Drawing for the job (mm, zero at the part's lowest x, y, z). Give positions to 0.01 mm unless a question says otherwise; leave off trailing zeros. Order: outer loops, then holes, each group sorted by start corner. A loop starts at its lowest first (then second) coordinate and runs counter-clockwise, first axis right, second up. Notation, with made-up numbers: (42.5, 48.5) - (66.5, 48.5) arc R15 ccw to (66.5, 52.5) - close; hole circle Ø7 at (-36, 44). An arc over 180 degrees is marked (long way). Use a Markdown table: item, result.
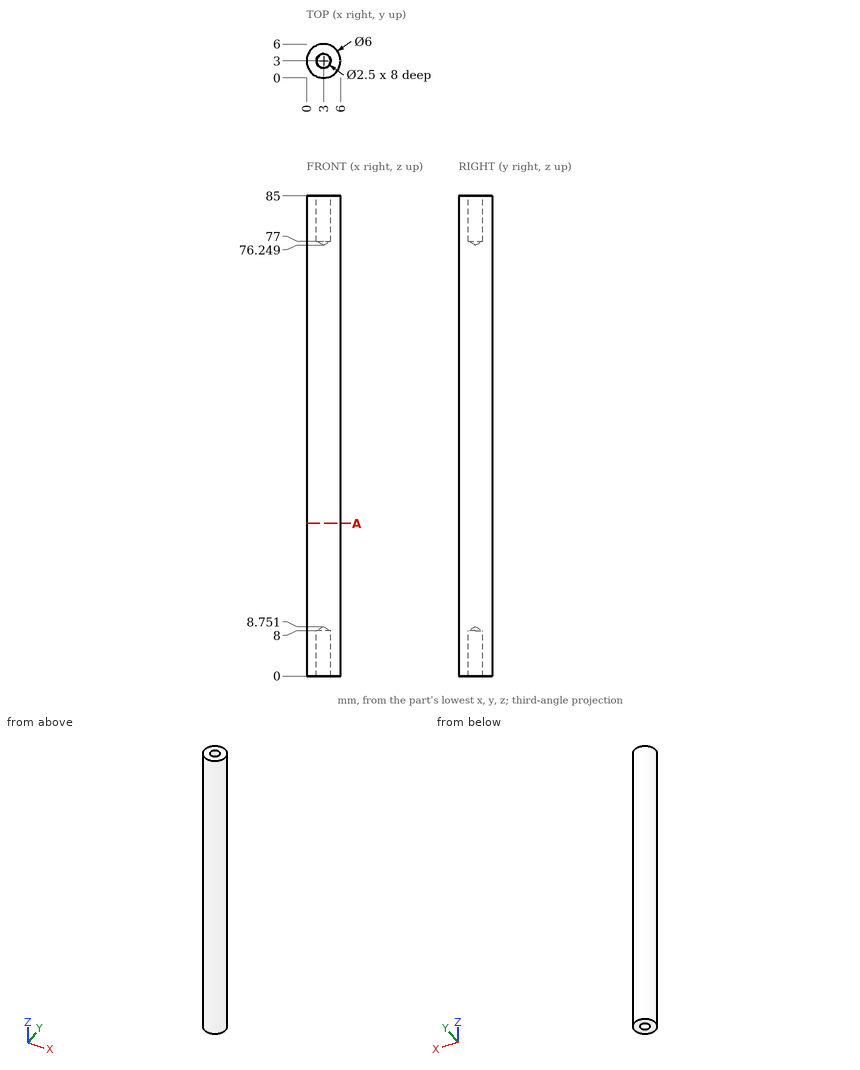
1) Wall check: line 1 (Y direction, x = 3, z = 4.25); line 2 (Y direction, x = 3.4, z = 54); line 3 (X direction, y = 4, z = 22). Give the ranges that are in metal, low to high. Write a range as from..to.
Computed:
| item | result |
|---|---|
| line 1 | y = 0..1.75, 4.25..6 |
| line 2 | y = 0.03..5.97 |
| line 3 | x = 0.17..5.83 |
2) Pin check, flat tips, straight feed: P1, Ø1.5, axis at x = 3, y = 3, coming from the +Z side; P2, Ø1.5, axis at x = 3, y = 3, coming from the -Z side; P3, Ø1, axis at y = 4, z = 25.5, coming from the -X side. Stop position of each tip, or through.
Computed:
| item | result |
|---|---|
| P1 | stops at z = 76.7 |
| P2 | stops at z = 8.3 |
| P3 | stops at x = 0.04 |
3) Slice it at A-A (z = 27). Write the cut outline in (x, y), and give its area (3 significant figures).
Computed:
| item | result |
|---|---|
| outline | circle Ø6 at (3, 3) |
| area | 28.3 mm² |
